Verification items for the finished model (mm, model axes). A direction names the side the tool comes from. Give positions to 0.01 mm unless a question says otherwise; leave off trailing zeros. Order: outer loops, then holes, each group sorted by start corner. A loop starts at its lowest first (then second) coordinate and runs counter-clockwise, first axis right, second up. Notation, with made-up numbers: (38, 69.5) - (54, 69.5) arc R37 ccw to (54, 106.5) - close; hole circle Ø1 at (-2, -34). An arc over 180 degrees is marked (long way). Answer as a JSON object with one key per item and string values.
```python
from build123d import *

# Parameters (mm, degrees)
ESBO_O1_W                = 25
ESBO_O1_H                = 51.5
RESSALTO_EXTRUS_O1_DEPTH = 1.5
ESBO_O4_W                = 25
ESBO_O4_H                = 1.5
RESSALTO_EXTRUS_O2_DEPTH = 25
ESBO_O5_R                = 1.65
ESBO_O5_R_2              = 3.7
CORTE_EXTRUS_O1_DEPTH    = 25
ESBO_O7_R                = 1.524
CORTE_EXTRUS_O2_DEPTH    = 25
FILETE1_R                = 5
FILETE2_R                = 2
FILETE3_R                = 1


with BuildPart() as part:
    # Esboço1 → Ressalto-extrusão1 (new body)
    with BuildSketch(Plane(origin=(0, 0, 0), x_dir=(1, 0, 0), z_dir=(0, 1, 0))):
        with Locations((12.5, 25.75)):
            Rectangle(ESBO_O1_W, ESBO_O1_H)
    extrude(amount=RESSALTO_EXTRUS_O1_DEPTH)

    # Esboço4 → Ressalto-extrusão2 (add)
    with BuildSketch(Plane(origin=(0, 1.5, 0), x_dir=(1, 0, 0), z_dir=(0, 1, 0))):
        with Locations((12.5, 0.75)):
            Rectangle(ESBO_O4_W, ESBO_O4_H)
    extrude(amount=RESSALTO_EXTRUS_O2_DEPTH)

    # Esboço5 → Corte-extrusão1 (cut)
    with BuildSketch(Plane.XY):
        with Locations((4, 14)):
            Circle(ESBO_O5_R)
        with BuildLine():
            ThreePointArc((0, 14), (3.661165235, 22.838834765), (12.5, 26.5))
            Line((12.5, 26.5), (0, 26.5))
            Line((0, 26.5), (0, 14))
        make_face()
        with Locations((12.5, 22.5)):
            Circle(ESBO_O5_R)
        with Locations((12.5, 14)):
            Circle(ESBO_O5_R_2)
        with Locations((21, 14)):
            Circle(ESBO_O5_R)
        with Locations((12.5, 5.5)):
            Circle(ESBO_O5_R)
        with BuildLine():
            ThreePointArc((12.5, 26.5), (21.338834765, 22.838834765), (25, 14))
            Line((25, 14), (25, 26.5))
            Line((25, 26.5), (12.5, 26.5))
        make_face()
    extrude(amount=-CORTE_EXTRUS_O1_DEPTH, mode=Mode.SUBTRACT)

    # Esboço7 → Corte-extrusão2 (cut)
    with BuildSketch(Plane(origin=(0, 1.5, 0), x_dir=(1, 0, 0), z_dir=(0, 1, 0))):
        with Locations((12.5, 40.68)):
            Circle(ESBO_O7_R)
        with Locations((12.5, 34.33)):
            Circle(ESBO_O7_R)
        with Locations((12.5, 27.98)):
            Circle(ESBO_O7_R)
        with Locations((12.5, 21.63)):
            Circle(ESBO_O7_R)
        with Locations((12.5, 15.28)):
            Circle(ESBO_O7_R)
        with Locations((12.5, 8.93)):
            Circle(ESBO_O7_R)
        with Locations((12.5, 47.08)):
            Circle(ESBO_O7_R)
        with BuildLine():
            Line((1.524, 3.956), (0.8, 3.956))
            ThreePointArc((0.8, 3.956), (0.234314575, 3.721685425), (0, 3.156))
            Line((0, 3.156), (0, 7.804))
            ThreePointArc((0, 7.804), (0.234314575, 7.238314575), (0.8, 7.004))
            Line((0.8, 7.004), (1.524, 7.004))
            ThreePointArc((1.524, 7.004), (3.048, 5.48), (1.524, 3.956))
        make_face()
        with BuildLine():
            Line((23.476, 45.404), (24.2, 45.404))
            ThreePointArc((24.2, 45.404), (24.765685425, 45.638314575), (25, 46.204))
            Line((25, 46.204), (25, 41.556))
            ThreePointArc((25, 41.556), (24.765685425, 42.121685425), (24.2, 42.356))
            Line((24.2, 42.356), (23.476, 42.356))
            ThreePointArc((23.476, 42.356), (21.952, 43.88), (23.476, 45.404))
        make_face()
        with BuildLine():
            Line((25, 35.156), (25, 39.804))
            ThreePointArc((25, 39.804), (24.765685425, 39.238314575), (24.2, 39.004))
            Line((24.2, 39.004), (23.476, 39.004))
            ThreePointArc((23.476, 39.004), (21.952, 37.48), (23.476, 35.956))
            Line((23.476, 35.956), (24.2, 35.956))
            ThreePointArc((24.2, 35.956), (24.765685425, 35.721685425), (25, 35.156))
        make_face()
        with BuildLine():
            Line((25, 28.756), (25, 33.404))
            ThreePointArc((25, 33.404), (24.765685425, 32.838314575), (24.2, 32.604))
            Line((24.2, 32.604), (23.476, 32.604))
            ThreePointArc((23.476, 32.604), (21.952, 31.08), (23.476, 29.556))
            Line((23.476, 29.556), (24.2, 29.556))
            ThreePointArc((24.2, 29.556), (24.765685425, 29.321685425), (25, 28.756))
        make_face()
        with BuildLine():
            Line((25, 22.356), (25, 27.004))
            ThreePointArc((25, 27.004), (24.765685425, 26.438314575), (24.2, 26.204))
            Line((24.2, 26.204), (23.476, 26.204))
            ThreePointArc((23.476, 26.204), (21.952, 24.68), (23.476, 23.156))
            Line((23.476, 23.156), (24.2, 23.156))
            ThreePointArc((24.2, 23.156), (24.765685425, 22.921685425), (25, 22.356))
        make_face()
        with BuildLine():
            Line((25, 15.956), (25, 20.604))
            ThreePointArc((25, 20.604), (24.765685425, 20.038314575), (24.2, 19.804))
            Line((24.2, 19.804), (23.476, 19.804))
            ThreePointArc((23.476, 19.804), (21.952, 18.28), (23.476, 16.756))
            Line((23.476, 16.756), (24.2, 16.756))
            ThreePointArc((24.2, 16.756), (24.765685425, 16.521685425), (25, 15.956))
        make_face()
        with BuildLine():
            Line((25, 9.556), (25, 14.204))
            ThreePointArc((25, 14.204), (24.765685425, 13.638314575), (24.2, 13.404))
            Line((24.2, 13.404), (23.476, 13.404))
            ThreePointArc((23.476, 13.404), (21.952, 11.88), (23.476, 10.356))
            Line((23.476, 10.356), (24.2, 10.356))
            ThreePointArc((24.2, 10.356), (24.765685425, 10.121685425), (25, 9.556))
        make_face()
        with BuildLine():
            Line((25, 3.156), (25, 7.804))
            ThreePointArc((25, 7.804), (24.765685425, 7.238314575), (24.2, 7.004))
            Line((24.2, 7.004), (23.476, 7.004))
            ThreePointArc((23.476, 7.004), (21.952, 5.48), (23.476, 3.956))
            Line((23.476, 3.956), (24.2, 3.956))
            ThreePointArc((24.2, 3.956), (24.765685425, 3.721685425), (25, 3.156))
        make_face()
        with BuildLine():
            Line((1.524, 10.356), (0.8, 10.356))
            ThreePointArc((0.8, 10.356), (0.234314575, 10.121685425), (0, 9.556))
            Line((0, 9.556), (0, 14.204))
            ThreePointArc((0, 14.204), (0.234314575, 13.638314575), (0.8, 13.404))
            Line((0.8, 13.404), (1.524, 13.404))
            ThreePointArc((1.524, 13.404), (3.048, 11.88), (1.524, 10.356))
        make_face()
        with BuildLine():
            Line((1.524, 16.756), (0.8, 16.756))
            ThreePointArc((0.8, 16.756), (0.234314575, 16.521685425), (0, 15.956))
            Line((0, 15.956), (0, 20.604))
            ThreePointArc((0, 20.604), (0.234314575, 20.038314575), (0.8, 19.804))
            Line((0.8, 19.804), (1.524, 19.804))
            ThreePointArc((1.524, 19.804), (3.048, 18.28), (1.524, 16.756))
        make_face()
        with BuildLine():
            Line((1.524, 23.156), (0.8, 23.156))
            ThreePointArc((0.8, 23.156), (0.234314575, 22.921685425), (0, 22.356))
            Line((0, 22.356), (0, 27.004))
            ThreePointArc((0, 27.004), (0.234314575, 26.438314575), (0.8, 26.204))
            Line((0.8, 26.204), (1.524, 26.204))
            ThreePointArc((1.524, 26.204), (3.048, 24.68), (1.524, 23.156))
        make_face()
        with BuildLine():
            Line((1.524, 29.556), (0.8, 29.556))
            ThreePointArc((0.8, 29.556), (0.234314575, 29.321685425), (0, 28.756))
            Line((0, 28.756), (0, 33.404))
            ThreePointArc((0, 33.404), (0.234314575, 32.838314575), (0.8, 32.604))
            Line((0.8, 32.604), (1.524, 32.604))
            ThreePointArc((1.524, 32.604), (3.048, 31.08), (1.524, 29.556))
        make_face()
        with BuildLine():
            Line((1.524, 35.956), (0.8, 35.956))
            ThreePointArc((0.8, 35.956), (0.234314575, 35.721685425), (0, 35.156))
            Line((0, 35.156), (0, 39.804))
            ThreePointArc((0, 39.804), (0.234314575, 39.238314575), (0.8, 39.004))
            Line((0.8, 39.004), (1.524, 39.004))
            ThreePointArc((1.524, 39.004), (3.048, 37.48), (1.524, 35.956))
        make_face()
        with BuildLine():
            Line((0, 41.556), (0, 46.204))
            ThreePointArc((0, 46.204), (0.234314575, 45.638314575), (0.8, 45.404))
            Line((0.8, 45.404), (1.524, 45.404))
            ThreePointArc((1.524, 45.404), (3.048, 43.88), (1.524, 42.356))
            Line((1.524, 42.356), (0.8, 42.356))
            ThreePointArc((0.8, 42.356), (0.234314575, 42.121685425), (0, 41.556))
        make_face()
    extrude(amount=-CORTE_EXTRUS_O2_DEPTH, mode=Mode.SUBTRACT)

    # Filete1
    filete1_edges = [part.edges().sort_by_distance(p)[0] for p in [
        (0, 0.75, -51.5),
        (25, 0.75, -51.5),
    ]]
    fillet(filete1_edges, radius=FILETE1_R)

    # Filete2
    filete2_edges = [part.edges().sort_by_distance(p)[0] for p in [
        (12.5, 0, 0),
    ]]
    fillet(filete2_edges, radius=FILETE2_R)

    # Filete3
    filete3_edges = [part.edges().sort_by_distance(p)[0] for p in [
        (12.5, 1.5, -1.5),
    ]]
    fillet(filete3_edges, radius=FILETE3_R)


solid = part.part
```
(1) Section check D-D (z = -11.88). Record the cut outline in (x, y), then the cut area to 3 significant figures.
Computed values:
{"outline": "(3.05, 0) - (21.95, 0) - (21.95, 1.5) - (3.05, 1.5) - close", "area": "28.4 mm²"}
(2) Section check B-B (x = 4). Record the cut outline in (y, z), then the cut area to 3 significant figures.
Computed values:
{"outline": "(0, -51.4) - (1.5, -51.4) - (1.5, -2.5) arc R1 cw to (2.5, -1.5) - (12.35, -1.5) - (12.35, 0) - (2, 0) arc R2 ccw to (0, -2) - close; (15.65, -1.5) - (23.17, -1.5) - (23.17, 0) - (15.65, 0) - close", "area": "104 mm²"}
(3) Release check for a two-part mould opening along Z. For faces 1 (the cylindrical face through (19.35, 14.07, -0.74)), 2 (the cylindrical face through (3.048, 0.76, -37.514)) record: pulls with the +Z half, pulls with the -Z half, needs draft (parallel to the pull), parting line crosses it, or undercut.
Computed values:
{"face 1": "needs draft", "face 2": "undercut"}
(4) Material ranges on line 1 along X through (y, z) = (0.5, -21.63); line 2 along Y through (x, z) = (12.5, -0.9); line 3 along Y through (x, z) = (17.25, -26), recorded low to high. Write a range as [from, to].
Computed values:
{"line 1": "x = [0, 10.98], [14.02, 25]", "line 2": "y = [0.33, 3.85], [7.15, 10.3], [17.7, 20.85], [24.15, 26.5]", "line 3": "y = [0, 1.5]"}
(5) Gauge pin test, flat ends, axial feed: pin 1 Ø0.8 at (x, y) = (1, 1) entering from +Z; pin 2 Ø1.8 at (x, z) = (12.5, -15.28) entering from +Y; pin 3 Ø6 at (x, y) = (17, 18) entering from -Z; pin 4 Ø4 at (x, z) = (15, -7.5) entering from +Y. Record the tip position at first contact, or that the pin passes through.
Computed values:
{"pin 1": "stops at z = -0.09", "pin 2": "passes through", "pin 3": "stops at z = -1.5", "pin 4": "stops at y = 1.5"}
(6) Section check A-A (z = -21.63). Record the cut outline in (x, y), then the cut area to 3 significant figures.
Computed values:
{"outline": "(0, 0) - (10.98, 0) - (10.98, 1.5) - (0, 1.5) - close; (14.02, 0) - (25, 0) - (25, 1.5) - (14.02, 1.5) - close", "area": "32.9 mm²"}
(7) Access from +Z, -Z, +X, -X, +Y, -Y to the whole of each face (thin tool, end or side, straight path). Record for faces 3 (the flat face through (25, 1, -41)), 4 (the flat face through (10, 1.5, -27)).
Computed values:
{"face 3": "+Z, -Z, +X, +Y, -Y", "face 4": "-Z, +X, -X, +Y"}
(8) Section check C-C (y = 22.5). Record the cut outline in (x, z), then the cut area to 3 significant figures.
Computed values:
{"outline": "(3.33, -1.5) - (10.85, -1.5) - (10.85, 0) - (3.33, 0) - close; (14.15, -1.5) - (21.67, -1.5) - (21.67, 0) - (14.15, 0) - close", "area": "22.5 mm²"}
